The figure shows three views and two pictorial views of one solid part (mm, origin at its lowest corner). Answer the questions. A direction names the side the tool comes from. Give positions to 0.01 mm unless a question says otherwise; leave off trailing zeros. Order: outer loops, then holes, each group sorted by start corner. A loop starts at its lowest first (then second) coordinate and runs counter-clockwise, first axis right, second up. Notation, with made-up numbers: (-24, 80.25) - (20, 80.25) arc R32 ccw to (20, 114.25) - close; hole circle Ø6 at (-6.75, 19.25). An arc over 180 degrees is marked (long way). Answer as a JSON object with one key per item and string values. Group by question number.
Q1. For the marked faces 1 and 2, determine the directions among +Z, -Z, +X, -X, +Y, -Y from which every point of the face is accessible in a straight line to the end or side of a thin tool.
Q2. A cutting plane is placed at C-C, the plane y = 39. Give the vertices of the cut face in (x, z) (1 decimal).
Q3. Consider line 1 (Y direction, x = 50, z = 12) (1 decimal); line 2 (X direction, y = 36.5, z = 1) (1 decimal); line 3 (Z direction, x = 71, y = 14). Determine where each line is inside the solid, lowest interval first.
Q4. A cutting plane is placed at A-A, the plane z = 8. Give the vertices of the cut face in (x, y) (1 decimal).
Q5. The mould has two halves that part along Y. Classify the marked faces 3, 4 and 5: released by +Y, released by -Y, zero draft, split by the parting line, or undercut.
Q6. Given pin 1 (4 mm diameter, centred on y = 3.5, z = 12, fed in from -X); pin 2 (12 mm diameter, centred on x = 49, y = 7.5, fed in from -Z), each flat-ended and moving along its own axis, determine where each tip first touches the part or whether it passes through.
Q7. A cutting plane is placed at B-B, the plane x = 43.5. Give the vertices of the cut face in (y, z) (1 decimal), and give its area (3 significant figures).
Q8. A cutting plane is placed at D-D, the plane x = 10. Give the vertices of the cut face in (y, z) (1 decimal), and give its area (3 significant figures).
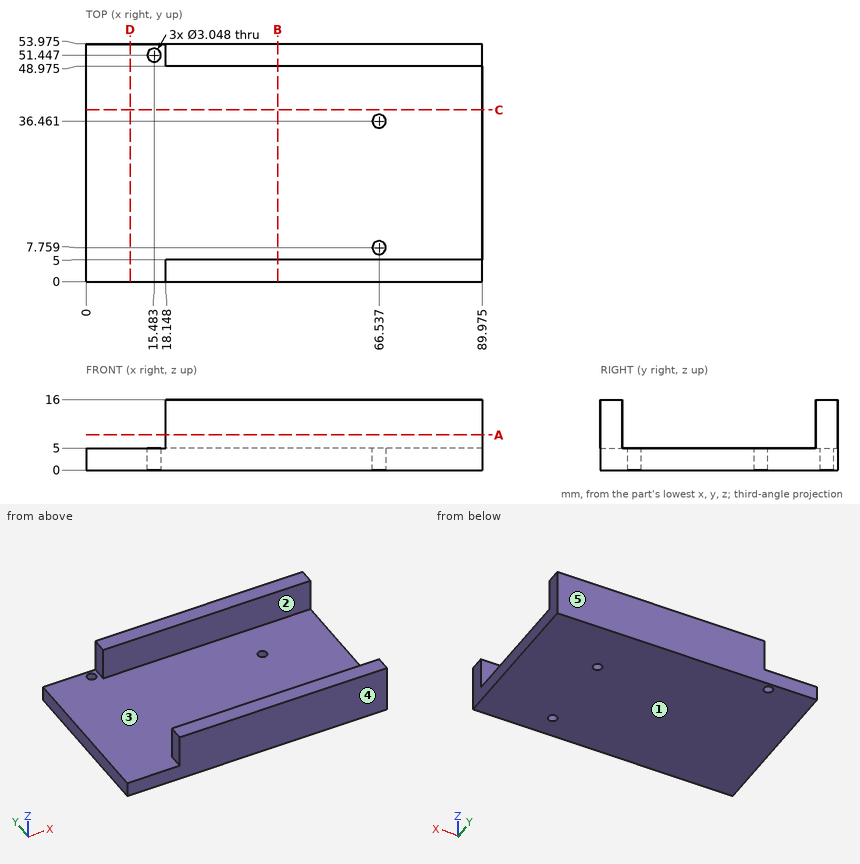
Reply:
{
 "1": {"face 1": "-Z, +X, -X, +Y, -Y", "face 2": "+Z, +X, -X"},
 "2": {"outline": "(0, 0) - (90, 0) - (90, 5) - (0, 5) - close"},
 "3": {"line 1": "y = 0 to 5, 49 to 54", "line 2": "x = 0 to 65, 68.1 to 90", "line 3": "z = 0 to 5"},
 "4": {"outline": "(18.1, 0) - (90, 0) - (90, 5) - (18.1, 5) - close; (18.1, 49) - (90, 49) - (90, 54) - (18.1, 54) - close"},
 "5": {"face 3": "undercut", "face 4": "released by -Y", "face 5": "released by +Y"},
 "6": {"pin 1": "stops at x = 18.15", "pin 2": "stops at z = 0"},
 "7": {"outline": "(0, 0) - (54, 0) - (54, 16) - (49, 16) - (49, 5) - (5, 5) - (5, 16) - (0, 16) - close", "area": "380 mm^2"},
 "8": {"outline": "(0, 0) - (54, 0) - (54, 5) - (0, 5) - close", "area": "270 mm^2"}
}
